```python
from build123d import *

# Parameters (mm, degrees)
SKETCH1_W           = 100
SKETCH1_H           = 48
BOSS_EXTRUDE1_DEPTH = 7
CUT_EXTRUDE1_REACH  = 113.144
SKETCH2_R           = 3.5
SKETCH3_W           = 100
SKETCH3_H           = 8
BOSS_EXTRUDE2_DEPTH = 10.2
SKETCH4_R           = 6.55
CUT_EXTRUDE2_DEPTH  = 5.25
SKETCH5_R           = 2.6
CUT_EXTRUDE3_DEPTH  = 7
SKETCH7_R           = 1.7
CUT_EXTRUDE4_DEPTH  = 112.391382072
CUT_EXTRUDE5_REACH  = 114.249
SKETCH8_R           = 1.7
SKETCH9_R           = 3
CUT_EXTRUDE6_DEPTH  = 10
FILLET1_R           = 20


with BuildPart() as part:
    # Sketch1 → Boss-Extrude1 (new body)
    with BuildSketch(Plane.XY):
        with Locations((50, 24)):
            Rectangle(SKETCH1_W, SKETCH1_H)
    extrude(amount=BOSS_EXTRUDE1_DEPTH)

    # Sketch2 → Cut-Extrude1 (cut, up to next)
    with BuildSketch(Plane.XY.offset(7), mode=Mode.PRIVATE) as cut_extrude1_sk1:
        with Locations((15, 29)):
            Circle(SKETCH2_R)
    cut_extrude1_tool1 = extrude(cut_extrude1_sk1.sketch, amount=-CUT_EXTRUDE1_REACH, mode=Mode.PRIVATE) & part.part
    # Sketch2 → Cut-Extrude1 (cut, up to next)
    with BuildSketch(Plane.XY.offset(7), mode=Mode.PRIVATE) as cut_extrude1_sk2:
        with Locations((33.75, 29)):
            Circle(SKETCH2_R)
    cut_extrude1_tool2 = extrude(cut_extrude1_sk2.sketch, amount=-CUT_EXTRUDE1_REACH, mode=Mode.PRIVATE) & part.part
    # Sketch2 → Cut-Extrude1 (cut, up to next)
    with BuildSketch(Plane.XY.offset(7), mode=Mode.PRIVATE) as cut_extrude1_sk3:
        with Locations((55, 29)):
            Circle(SKETCH2_R)
    cut_extrude1_tool3 = extrude(cut_extrude1_sk3.sketch, amount=-CUT_EXTRUDE1_REACH, mode=Mode.PRIVATE) & part.part
    # Sketch2 → Cut-Extrude1 (cut, up to next)
    with BuildSketch(Plane.XY.offset(7), mode=Mode.PRIVATE) as cut_extrude1_sk4:
        with Locations((76.25, 29)):
            Circle(SKETCH2_R)
    cut_extrude1_tool4 = extrude(cut_extrude1_sk4.sketch, amount=-CUT_EXTRUDE1_REACH, mode=Mode.PRIVATE) & part.part
    add(cut_extrude1_tool1.solids().sort_by_distance((15, 29, 7))[0], mode=Mode.SUBTRACT)
    add(cut_extrude1_tool2.solids().sort_by_distance((33.75, 29, 7))[0], mode=Mode.SUBTRACT)
    add(cut_extrude1_tool3.solids().sort_by_distance((55, 29, 7))[0], mode=Mode.SUBTRACT)
    add(cut_extrude1_tool4.solids().sort_by_distance((76.25, 29, 7))[0], mode=Mode.SUBTRACT)

    # Sketch3 → Boss-Extrude2 (add)
    with BuildSketch(Plane(origin=(0, 0, 0), x_dir=(-1, 0, 0), z_dir=(0, 0, -1))):
        with Locations((-50, 4)):
            Rectangle(SKETCH3_W, SKETCH3_H)
    extrude(amount=BOSS_EXTRUDE2_DEPTH)

    # Sketch4 → Cut-Extrude2 (cut)
    with BuildSketch(Plane(origin=(0, 0, 0), x_dir=(-1, 0, 0), z_dir=(0, 0, -1))):
        with Locations((-76.25, 29)):
            Circle(SKETCH4_R)
        with Locations((-55, 29)):
            Circle(SKETCH4_R)
        with Locations((-33.75, 29)):
            Circle(SKETCH4_R)
        with Locations((-15, 29)):
            Circle(SKETCH4_R)
    extrude(amount=-CUT_EXTRUDE2_DEPTH, mode=Mode.SUBTRACT)

    # Sketch5 → Cut-Extrude3 (cut)
    with BuildSketch(Plane.XY.offset(7)):
        with Locations((35.000022648, 4.052132501)):
            Circle(SKETCH5_R)
        with Locations((64.999977352, 4)):
            Circle(SKETCH5_R)
    extrude(amount=-CUT_EXTRUDE3_DEPTH, mode=Mode.SUBTRACT)

    # Sketch7 → Cut-Extrude4 (cut, through all)
    with BuildSketch(Plane.XY):
        with Locations((35.000022648, 4.052132501)):
            Circle(SKETCH7_R)
        with Locations((64.999977352, 4)):
            Circle(SKETCH7_R)
    extrude(amount=-CUT_EXTRUDE4_DEPTH, mode=Mode.SUBTRACT)

    # Sketch8 → Cut-Extrude5 (cut, up to next)
    with BuildSketch(Plane.XY.offset(7), mode=Mode.PRIVATE) as cut_extrude5_sk1:
        with Locations((10, 4.052132501)):
            Circle(SKETCH8_R)
    cut_extrude5_tool1 = extrude(cut_extrude5_sk1.sketch, amount=-CUT_EXTRUDE5_REACH, mode=Mode.PRIVATE) & part.part
    # Sketch8 → Cut-Extrude5 (cut, up to next)
    with BuildSketch(Plane.XY.offset(7), mode=Mode.PRIVATE) as cut_extrude5_sk2:
        with Locations((90, 4.052132501)):
            Circle(SKETCH8_R)
    cut_extrude5_tool2 = extrude(cut_extrude5_sk2.sketch, amount=-CUT_EXTRUDE5_REACH, mode=Mode.PRIVATE) & part.part
    add(cut_extrude5_tool1.solids().sort_by_distance((10, 4.052133, 7))[0], mode=Mode.SUBTRACT)
    add(cut_extrude5_tool2.solids().sort_by_distance((90, 4.052133, 7))[0], mode=Mode.SUBTRACT)

    # Sketch9 → Cut-Extrude6 (cut)
    with BuildSketch(Plane.XY.offset(7)):
        with Locations((10, 4.052132501)):
            Circle(SKETCH9_R)
        with Locations((90, 4.052132501)):
            Circle(SKETCH9_R)
    extrude(amount=-CUT_EXTRUDE6_DEPTH, mode=Mode.SUBTRACT)

    # Fillet1
    fillet1_edges = [part.edges().sort_by_distance(p)[0] for p in [
        (0, 48, 3.5),
        (100, 48, 3.5),
    ]]
    fillet(fillet1_edges, radius=FILLET1_R)


solid = part.part
```
Part model, mm, in its own coordinate system. A direction names the side the tool comes from. Round coordinates to 2 decimals unless told otherwise and drop trailing zeros. Order: outer loops, then holes, each group sorted by start corner. A loop starts at its lowest first (then second) coordinate and runs counter-clockwise, first axis right, second up. Notation, with made-up numbers: M -17.75,-18 L 7.25,-18 A22 cw 7.25,0 Z; hole C -33,2 d6. An arc over 180 degrees is marked long. Answer in a Markdown table with one row per item. Add a question column.
Q1. Mould opens along Y. For faces 4 (the face through (49, 24, 0)), 5 (the face through (31, 26, 5.25)), 6 (the face through (94.297, 41.986, 3.549)), 7 (the face through (51, 0, -1)) say: +Y half, -Y half, draft (parallel to the pull), parting line (faces both ways), or undercut.
Q2. Cut at D-D on y = 29. Give the number of separate pieces and of enclosed holes in the cut face, and give its area (3 significant figures).
Q3. Pin check, flat tips, straight feed: pin 1 (8 mm diameter, centred on x = 15, y = 29, fed in from -Z); pin 2 (5 mm diameter, centred on x = 75, z = -6.5, fed in from +Y); pin 3 (1.8 mm diameter, centred on x = 89, y = 4.5, fed in from +Z). Stop position of each tip, or through.
Q4. 3-axis set-ups, long thin cutter, end or side, ignore diameter. For faces 1 (the face through (0, 10.7, 0.4)), 2 (the face through (36, 2, 0)), 3 (the face through (56.4, 22.6, 2.6)): which of +Z, -Z, +X, -X, +Y, -Y reach the whole face in a straight line?
Q5. Cut at C-C on x = 45. Give the cut face in (y, z).
Q6. Cut at A-A on x = 55. Give the cut face in (y, z), and give its area (3 significant figures).
Q7. Wall check: L1, parallel to Y at x = 90, z = -1; L2, parallel to X at y = 30.5, z = 1.75; L3, parallel to X at y = 3, z = -7.5. Give the ranges that are in metal, low to high. Write a range as from..to.
Q8. Cut at B-B on x = 35. Give the cut face in (y, z), and give its area (3 significant figures).
Established:
| question | item | result |
|---|---|---|
| 1 | face 4 | draft |
| 1 | face 5 | undercut |
| 1 | face 6 | +Y half |
| 1 | face 7 | -Y half |
| 2 | separate pieces | 5 |
| 2 | enclosed holes | 0 |
| 2 | area | 376 mm2 |
| 3 | pin 1 | stops at z = 5.25 |
| 3 | pin 2 | stops at y = 8 |
| 3 | pin 3 | stops at z = -3 |
| 4 | face 1 | +Z, -Z, -X, +Y, -Y |
| 4 | face 2 | +Z |
| 4 | face 3 | -Z |
| 5 | outline | M 0,-10.2 L 8,-10.2 L 8,0 L 48,0 L 48,7 L 0,7 Z |
| 6 | outline | M 0,-10.2 L 8,-10.2 L 8,0 L 22.45,0 L 22.45,5.25 L 25.5,5.25 L 25.5,7 L 0,7 Z; M 32.5,5.25 L 35.55,5.25 L 35.55,0 L 48,0 L 48,7 L 32.5,7 Z |
| 6 | area | 337 mm2 |
| 7 | L1 | y = 0..1.05, 7.05..8 |
| 7 | L2 | x = 0.16..8.62, 21.38..27.37, 40.13..48.62, 61.38..69.87, 82.63..99.84 |
| 7 | L3 | x = 0..8.66, 11.34..33.66, 36.34..63.63, 66.37..88.66, 91.34..100 |
| 8 | outline | M 0,-10.2 L 2.35,-10.2 L 2.35,0 L 1.45,0 L 1.45,7 L 0,7 Z; M 5.75,-10.2 L 8,-10.2 L 8,0 L 22.57,0 L 22.57,5.25 L 25.73,5.25 L 25.73,7 L 6.65,7 L 6.65,0 L 5.75,0 Z; M 32.27,5.25 L 35.43,5.25 L 35.43,0 L 48,0 L 48,7 L 32.27,7 Z |
| 8 | area | 268 mm2 |
